For this review, use the dimensioned drawing (mm, ordinates from the lowest corner) and the shaded views. A direction names the side the tool comes from. Coordinates: 2 decimals unless noted, no trailing zeros. Write each loop counter-clockwise with the first axis right and the second up, starting at its lowest first coordinate (ties: lowest second). Pieces come first, ordered by that corner, then holes. Notation, with made-up numbers: (68, -22) -> (78, -22) arc R33 ccw to (78, 7) -> close; hole circle Ø10 at (49.5, 10). An arc over 180 degrees is marked (long way). Put each result on its own line as item: value. Start each with the question number.
Item 1: Consider section C-C on z = 54. Give the boundary of the cut face in (x, y), and give its area (3 significant figures).
Item 2: To check wall thickness, follow L1, parallel to Z at x = 73.5, y = 27; L2, parallel to X at y = 27, z = 9.5; L3, parallel to X at y = 28.5, z = 85.5. State the ranges of each line that lie inside material, in increasing order.
Item 3: For the marked faces 1 and 2, list the 3-axis set-ups (+Z, -Z, +X, -X, +Y, -Y) from which the entire face can be reached by the end or side of a thin tool; tool diameter is ignored.
Item 4: Insertion check: P1, Ø4, axis at y = 42, z = 56.5, coming from the -X side; P2, Ø1.5, axis at y = 32, z = 83.5, coming from the -X side; P3, Ø3, axis at y = 53.5, z = 50, coming from the +X side; P4, Ø4, axis at x = 53, y = 37, coming from the -Z side. Each pin has a flat end and moves straight along its axis. Give the tip position at first contact, or say it passes through.
Item 5: Consider section D-D on x = 52.5. Give the boundary of the cut face in (y, z).
Item 6: Consider section A-A on x = 38.1. Give the boundary of the cut face in (y, z).
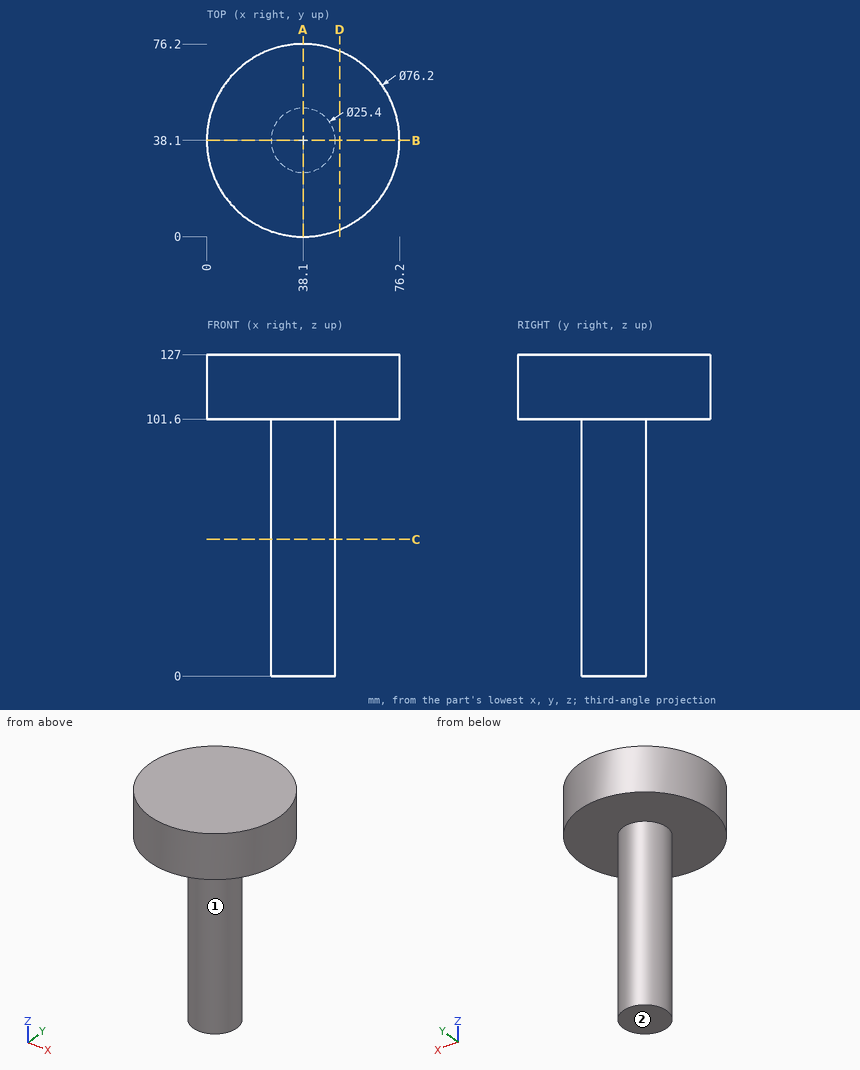
Return value:
1. outline: circle Ø25.4 at (38.1, 38.1)
1. area: 507 mm^2
2. L1: 101.6 to 127
2. L2: 31.93 to 44.27
2. L3: 29.79 to 46.41
3. face 1: -Z
3. face 2: -Z, +X, -X, +Y, -Y
4. P1: x = 25.54
4. P2: x = 26.58
4. P3: through
4. P4: z = 101.6
5. outline: (2.83, 101.6) -> (73.37, 101.6) -> (73.37, 127) -> (2.83, 127) -> close
6. outline: (0, 101.6) -> (25.4, 101.6) -> (25.4, 0) -> (50.8, 0) -> (50.8, 101.6) -> (76.2, 101.6) -> (76.2, 127) -> (0, 127) -> close
